```python
from build123d import *

# Parameters (mm, degrees)
F1_DEPTH = 1.5
F3_R     = 2


with BuildPart() as f1:
    # F0 (on Front) → F1 (new body, symmetric)
    with BuildSketch(Plane.XZ):
        Polygon((0, 47), (0, 172), (-73, 172), (-73, 0), (-31, 0), (-31, 47), align=None)
    extrude(amount=F1_DEPTH, both=True)

    # F2: F1 across plane


with BuildPart() as f1_1:
    add(f1.part)
    add(f1.part.mirror(Plane.YZ))

    # F3
    f3_edges = [f1_1.edges().sort_by_distance(p)[0] for p in [
        (73, 0, 172),
        (-73, 0, 172),
        (-31, 0, 0),
        (-73, 0, 0),
        (-31, 0, 47),
        (31, 0, 0),
        (31, 0, 47),
        (73, 0, 0),
    ]]
    fillet(f3_edges, radius=F3_R)


solid = f1_1.part
```
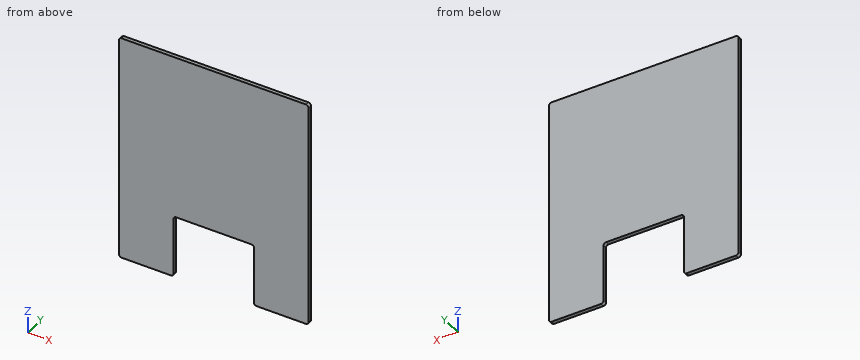
Source: CAD feature listing. Evaluate the final solid. Frame: model axes, mm. Give positions to 0.01 mm unless a question says otherwise; leave off trailing zeros. Loops run counter-clockwise (first coordinate to the right, second up) from the corner with the lowest first, then second, coordinate; pieces in that order, holes last. Notation, with made-up numbers: (-23, -20) - (5, -20) arc R14 ccw to (5, -9) - close; hole circle Ø9 at (8, -13). An arc over 180 degrees is marked (long way). Use CSV: the item, a comma, the result in double quotes. Start each with the question number.
1. Section B-B (y = 0). Output: boundary loops of the cut face in (x, z), then the cut area to 3 significant figures.
2. Section C-C (x = -19). Output: boundary loops of the cut face in (y, z).
3. Ray query, L1, parallel to X at y = 0.55, z = 13; L2, parallel to Z at x = -25.5, y = 1; L3, parallel to Z at x = -32, y = -1.35. Return the intervals inside material, ascending.
4. Section A-A (z = 34). Output: boundary loops of the cut face in (x, y), then the cut area to 3 significant figures.
5. Pin query (flat end, axial travel): pin 1 (1.5 mm diameter, centred on x = -5, y = 0.5, fed in from -Z). Return the tip coordinate at first contact, or that it passes through.
Response:
1,outline,"(-73, 2) arc R2 ccw to (-71, 0) - (-33, 0) arc R2 ccw to (-31, 2) - (-31, 45) arc R2 cw to (-29, 47) - (29, 47) arc R2 cw to (31, 45) - (31, 2) arc R2 ccw to (33, 0) - (71, 0) arc R2 ccw to (73, 2) - (73, 170) arc R2 ccw to (71, 172) - (-71, 172) arc R2 ccw to (-73, 170) - close"
1,area,"22,200 mm²"
2,outline,"(-1.5, 47) - (1.5, 47) - (1.5, 172) - (-1.5, 172) - close"
3,L1,"-73 to -31, 31 to 73"
3,L2,"47 to 172"
3,L3,"0.27 to 172"
4,outline,"(-73, -1.5) - (-31, -1.5) - (-31, 1.5) - (-73, 1.5) - close; (31, -1.5) - (73, -1.5) - (73, 1.5) - (31, 1.5) - close"
4,area,"252 mm²"
5,pin 1,"z = 47"
